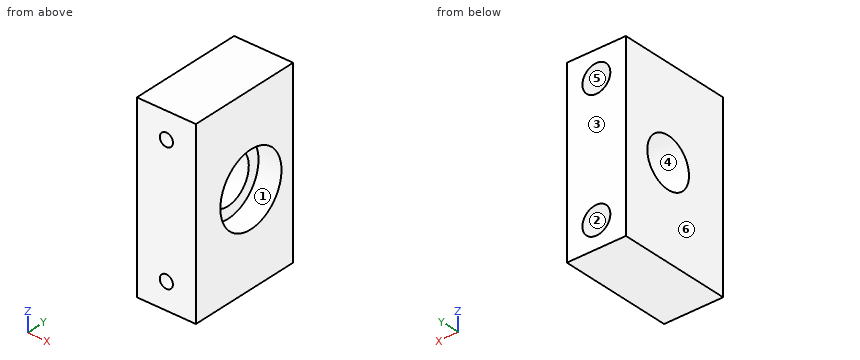
```python
from build123d import *

# Parameters (mm, degrees)
ESQUISSE1_W             = 55
ESQUISSE1_H             = 35
BOSS_EXTRU_1_DEPTH      = 18
ESQUISSE2_R             = 11
ENL_V_MAT_EXTRU_1_DEPTH = 7
ESQUISSE3_R             = 7.5
ENL_V_MAT_EXTRU_2_DEPTH = 302.152136256
ESQUISSE4_R             = 2
ENL_V_MAT_EXTRU_3_DEPTH = 299.279472876
ESQUISSE5_R             = 4.25
ENL_V_MAT_EXTRU_4_DEPTH = 12


with BuildPart() as part:
    # Esquisse1 → Boss.-Extru.1 (new body)
    with BuildSketch(Plane(origin=(0, 0, 0), x_dir=(0, 0, -1), z_dir=(1, 0, 0))):
        with Locations((-268.171513574, -36.785957969)):
            Rectangle(ESQUISSE1_W, ESQUISSE1_H)
    extrude(amount=BOSS_EXTRU_1_DEPTH)

    # Esquisse2 → Enlèv. mat.-Extru.1 (cut)
    with BuildSketch(Plane(origin=(18, 0, 0), x_dir=(0, 0, -1), z_dir=(1, 0, 0))):
        with Locations((-268.171513574, -34.485781453)):
            Circle(ESQUISSE2_R)
    extrude(amount=-ENL_V_MAT_EXTRU_1_DEPTH, mode=Mode.SUBTRACT)

    # Esquisse3 → Enlèv. mat.-Extru.2 (cut, through all)
    with BuildSketch(Plane.ZY):
        with Locations((268.171513574, -34.485781453)):
            Circle(ESQUISSE3_R)
    extrude(amount=-ENL_V_MAT_EXTRU_2_DEPTH, mode=Mode.SUBTRACT)

    # Esquisse4 → Enlèv. mat.-Extru.3 (cut, through all)
    with BuildSketch(Plane(origin=(0, -19.285957969, 0), x_dir=(1, 0, 0), z_dir=(0, 1, 0))):
        with Locations(Location((9, -287.671513574, 0), (0, 0, 270))):
            Circle(ESQUISSE4_R)
        with Locations(Location((9, -248.671513574, 0), (0, 0, 270))):
            Circle(ESQUISSE4_R)
    extrude(amount=-ENL_V_MAT_EXTRU_3_DEPTH, mode=Mode.SUBTRACT)

    # Esquisse5 → Enlèv. mat.-Extru.4 (cut)
    with BuildSketch(Plane(origin=(0, -19.285957969, 0), x_dir=(1, 0, 0), z_dir=(0, 1, 0))):
        with Locations(Location((9, -287.671513574, 0), (0, 0, 270))):
            Circle(ESQUISSE5_R)
        with Locations(Location((9, -248.671513574, 0), (0, 0, 270))):
            Circle(ESQUISSE5_R)
    extrude(amount=-ENL_V_MAT_EXTRU_4_DEPTH, mode=Mode.SUBTRACT)


solid = part.part
```
Part model, mm, in its own coordinate system. Face numbers are marked on the shaded views. A direction names the side the tool comes from. Round coordinates to 2 decimals unless told otherwise and drop trailing zeros. Loops run counter-clockwise (first coordinate to the right, second up) from the corner with the lowest first, then second, coordinate; pieces in that order, holes last.
1. Slice it at D-D (y = -50.5). Give the cut face in (x, z), and give its area (3 significant figures).
Solutions:
outline: (0, 240.67) - (18, 240.67) - (18, 295.67) - (0, 295.67) - close; hole circle Ø4 at (9, 248.67); hole circle Ø4 at (9, 287.67)
area: 965 mm2
2. Drill centre lines: line 1 along Y through (x, z) = (2.25, 268); line 2 along Z through (x, y) = (8.75, -33); line 3 along Z through (x, y) = (10.5, -40). Where is each one in solid material? Low to high.
Solutions:
line 1: y = -54.29 to -41.98, -26.99 to -19.29
line 2: z = 240.67 to 246.69, 250.66 to 260.82, 275.52 to 285.69, 289.66 to 295.67
line 3: z = 240.67 to 247.35, 249.99 to 263.09, 273.26 to 286.35, 288.99 to 295.67
3. 3-axis set-ups, long thin cutter, end or side, ignore diameter. For the marked faces 5 and 6: which of +Z, -Z, +X, -X, +Y, -Y reach the whole face in a straight line?
Solutions:
face 5: +Y
face 6: +Z, -Z, -X, +Y, -Y
4. Slice it at A-A (x = 9.75). Give the cut face in (y, z), and give its area (3 significant figures).
Solutions:
outline: (-54.29, 240.67) - (-19.29, 240.67) - (-19.29, 244.49) - (-31.29, 244.49) - (-31.29, 246.82) - (-54.29, 246.82) - close; (-54.29, 250.53) - (-31.29, 250.53) - (-31.29, 252.85) - (-19.29, 252.85) - (-19.29, 283.49) - (-31.29, 283.49) - (-31.29, 285.82) - (-54.29, 285.82) - close; (-54.29, 289.53) - (-31.29, 289.53) - (-31.29, 291.85) - (-19.29, 291.85) - (-19.29, 295.67) - (-54.29, 295.67) - close; hole circle Ø15 at (-34.49, 268.17)
area: 1,380 mm2
5. Flat gauge pins, fed straight in: pin 1 (2 mm diameter, centred on y = -26, z = 273, fed in from +X); pin 2 (5 mm diameter, centred on y = -39.5, z = 259.5, fed in from +X); pin 3 (5 mm diameter, centred on x = 9, z = 248.67, fed in from +Y). Where does each tip first touch, or does it go through?
Solutions:
pin 1: stops at x = 11
pin 2: stops at x = 18
pin 3: stops at y = -31.29
6. Two-plate mould, pull along Y, no slides. Class the marked faces 1, 2, 3 and 4: pulls with the +Y half, pulls with the -Y half, needs draft (parallel to the pull), parting line crosses it, or undercut.
Solutions:
face 1: undercut
face 2: needs draft
face 3: pulls with the +Y half
face 4: undercut
7. Slice it at B-B (y = -32). Give the cut face in (x, z).
Solutions:
outline: (0, 240.67) - (18, 240.67) - (18, 257.46) - (11, 257.46) - (11, 261.1) - (0, 261.1) - close; (0, 275.25) - (11, 275.25) - (11, 278.89) - (18, 278.89) - (18, 295.67) - (0, 295.67) - close; hole circle Ø4 at (9, 248.67); hole circle Ø4 at (9, 287.67)
8. Slice it at C-C (z = 274). Give the cut face in (x, y), and give its area (3 significant figures).
Solutions:
outline: (0, -54.29) - (18, -54.29) - (18, -43.81) - (11, -43.81) - (11, -39.21) - (0, -39.21) - close; (0, -29.77) - (11, -29.77) - (11, -25.16) - (18, -25.16) - (18, -19.29) - (0, -19.29) - close
area: 396 mm2
